Verification items for the finished model (mm, model axes). A direction names the side the tool comes from. Give positions to 0.01 mm unless a question says otherwise; leave off trailing zeros. Order: outer loops, then holes, each group sorted by start corner. A loop starts at its lowest first (then second) coordinate and runs counter-clockwise, first axis right, second up. Notation, with made-up numbers: (-25, -22.75) - (4, -22.75) arc R26 ccw to (4, 1.25) - close; hole circle Ø1 at (36, 84). An arc over 180 degrees is marked (long way). Answer as a JSON object with one key per item and string values. Group by question number.
(1) Access from +Z, -Z, +X, -X, +Y, -Y to the whole of each face (thin tool, end or side, straight path). Record for faces 1 (the face through (1, 3, -13)), 2 (the face through (-7.1, 4.3, -6)), 3 (the face through (-11.016, 4.837, -12.424)).
(2) Depth check by flat-ended pin: pin 1 Ø5 at (y, z) = (-1, -13.5) entering from -X; pin 2 Ø6 at (y, z) = (3.5, -9.5) entering from +X; pin 3 Ø1.5 at (x, z) = (-12, -9) entering from +Y; pin 4 Ø4 at (x, y) = (-12.5, -1.5) entering from -Z. Enter the tip coordinate at first touch or a pass-through.
(3) Section check D-D (y = -4). Record the boundary of the cut face in (x, z).
(4) Section check C-C (z = -12.5). Record the boundary of the cut face in (x, y), then the cut area to 3 significant figures.
(5) Thickness scan on line 1 (X direction, y = 2.75, z = -10); line 2 (X direction, y = 1.5, z = -12.75); line 3 (Z direction, x = -14.5, y = 1.5). Record the ranges inside material, lowest first.
(6) Section check A-A (y = 0). Record the boundary of the cut face in (x, z), then the cut area to 3 significant figures.
(7) Section check B-B (x = -7). Record the boundary of the cut face in (y, z), then the cut area to 3 significant figures.
```python
from build123d import *

# Parameters (mm, degrees)
BOX004_W           = 19
BOX004_H           = 20
BOX004_DEPTH       = 4
CYLINDER002_R      = 12.5
CYLINDER002_DEPTH  = 5
CYLINDER001_R      = 13
CYLINDER001_DEPTH  = 10
POCKET004012_DEPTH = 10


with BuildPart() as box004:
    # Box004 → Box004 (new body)
    with BuildSketch(Plane(origin=(-11, -12, -17), x_dir=(1, 0, 0), z_dir=(0, 0, 1))):
        with Locations((9.5, 10)):
            Rectangle(BOX004_W, BOX004_H)
    extrude(amount=BOX004_DEPTH)


with BuildPart() as cylinder002:
    # Cylinder002 → Cylinder002 (new body)
    with BuildSketch(Plane(origin=(-7, -7, -16), x_dir=(1, 0, 0), z_dir=(0, 0, 1))):
        Circle(CYLINDER002_R)
    extrude(amount=CYLINDER002_DEPTH)


with BuildPart() as cut002:
    # Cylinder001 → Cylinder001 (new body)
    with BuildSketch(Plane(origin=(-7, -7, -16), x_dir=(1, 0, 0), z_dir=(0, 0, 1))):
        Circle(CYLINDER001_R)
    extrude(amount=CYLINDER001_DEPTH)

    # Sketch020 → Pocket004012 (cut)
    with BuildSketch(Plane(origin=(-7, -7, -6), x_dir=(1, 0, 0), z_dir=(0, 0, 1))):
        with BuildLine():
            ThreePointArc((11.043126, 0), (0, 11.043126), (-11.043126, 0))
            Line((-11.043126, 0), (-15.353921, 0))
            Line((-15.353921, 0), (-15.353921, -14.225527))
            Line((-15.353921, -14.225527), (14.925669, -14.225527))
            Line((14.925669, -14.225527), (14.925669, 0))
            Line((14.925669, 0), (11.043126, 0))
        make_face()
    extrude(amount=-POCKET004012_DEPTH, mode=Mode.SUBTRACT)

    # Cut001: cut Cylinder002
    add(cylinder002.part, mode=Mode.SUBTRACT)

    # Cut002: cut Box004
    add(box004.part, mode=Mode.SUBTRACT)


solid = cut002.part
```
Solutions:
{
 "1": {"face 1": "-Z, +X, +Y, -Y", "face 2": "+Z, +X, -X, +Y, -Y", "face 3": "-Z, -Y"},
 "2": {"pin 1": "stops at x = -19.52", "pin 2": "stops at x = 3.62", "pin 3": "stops at y = 5.29", "pin 4": "passes through"},
 "3": {"outline": "(-19.65, -16) - (-19.13, -16) - (-19.13, -11) - (-17.63, -11) - (-17.63, -6) - (-19.65, -6) - close; (3.63, -11) - (5.13, -11) - (5.13, -13) - (5.65, -13) - (5.65, -6) - (3.63, -6) - close"},
 "4": {"outline": "(-20, -7) - (-19.5, -7) arc R12.5 cw to (5.5, -7) - (6, -7) arc R13 ccw to start", "area": "20.0 mm2"},
 "5": {"line 1": "x = -15.6 to -12.19, -1.81 to 1.6", "line 2": "x = -16.84 to -16.17, 2.17 to 2.84", "line 3": "z = -11 to -6"},
 "6": {"outline": "(-17.95, -16) - (-17.36, -16) - (-17.36, -11) - (-15.54, -11) - (-15.54, -6) - (-17.95, -6) - close; (1.54, -11) - (3.36, -11) - (3.36, -13) - (3.95, -13) - (3.95, -6) - (1.54, -6) - close", "area": "28.3 mm2"},
 "7": {"outline": "(4.04, -11) - (5.5, -11) - (5.5, -13) - (6, -13) - (6, -6) - (4.04, -6) - close", "area": "10.8 mm2"}
}
